Geometry: see drawing. Coordinates: mm, zero at the bounding-box minimum. A direction names the side the tool comes from. Round coordinates to 2 decimals unless told otherwise and drop trailing zeros. Loops run counter-clockwise (first coordinate to the right, second up) from the corner with the lowest first, then second, coordinate; pieces in that order, holes last. Notation, with made-up numbers: (57, 76.5) - (82, 76.5) arc R31 ccw to (82, 109.5) - close; hole circle Ø1 at (28, 13). An arc over 180 degrees is marked (long way). Return JSON: item names as keys, results as strings. Group by question number.
1. Section C-C on x = 65. Return loops of the section in (y, z), and give its area (3 significant figures).
2. First-contact query: pin 1 Ø4 at (x, y) = (44.5, 45) entering from -Z. Flat tip, straight axial feed; report the tip coordinate or a pass-through.
3. Section B-B on y = 10. Return loops of the section in (x, z).
4. Section D-D on y = 44. Return loops of the section in (x, z), and give its area (3 significant figures).
5. Set-up query: the marked faces 1 and 2. Return all of +Z, -Z, +X, -X, +Y, -Y with unobstructed straight access to the full face (end or side cutting, diameter ignored); none if empty.
6. Section A-A on z = 65. Return loops of the section in (x, y), and give its area (3 significant figures).
7. Material intervals for probe 1 along Y at (x, z) = (65, 85); probe 2 along Z at (x, y) = (95, 10); probe 3 along X at (y, z) = (30, 85.5), sorted ascending.
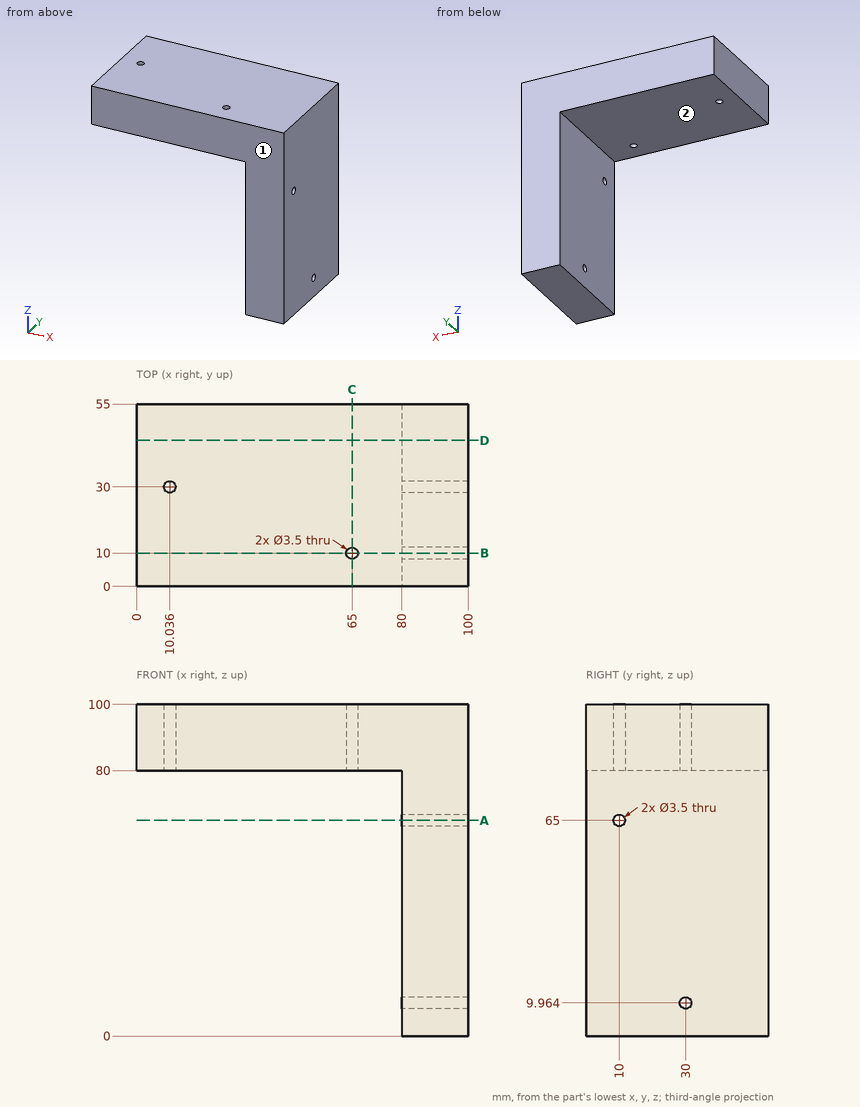
Taken from the geometry:
{
 "1": {"outline": "(0, 80) - (8.25, 80) - (8.25, 100) - (0, 100) - close; (11.75, 80) - (55, 80) - (55, 100) - (11.75, 100) - close", "area": "1,030 mm2"},
 "2": {"pin 1": "z = 80"},
 "3": {"outline": "(0, 80) - (63.25, 80) - (63.25, 100) - (0, 100) - close; (66.75, 80) - (80, 80) - (80, 66.75) - (100, 66.75) - (100, 100) - (66.75, 100) - close; (80, 0) - (100, 0) - (100, 63.25) - (80, 63.25) - close"},
 "4": {"outline": "(0, 80) - (80, 80) - (80, 0) - (100, 0) - (100, 100) - (0, 100) - close", "area": "3,600 mm2"},
 "5": {"face 1": "+Z, -Z, +X, -X, -Y", "face 2": "-Z, -X, +Y, -Y"},
 "6": {"outline": "(80, 0) - (100, 0) - (100, 8.25) - (80, 8.25) - close; (80, 11.75) - (100, 11.75) - (100, 55) - (80, 55) - close", "area": "1,030 mm2"},
 "7": {"probe 1": "0 to 8.25, 11.75 to 55", "probe 2": "0 to 63.25, 66.75 to 100", "probe 3": "0 to 8.29, 11.79 to 100"}
}
